Input: part model. Units: mm. Frame: model coordinates. Face numbers are marked on the shaded views. Coordinates: 2 decimals unless noted, no trailing zeros. Order: outer loops, then holes, each group sorted by start corner. A loop starts at its lowest first (then second) coordinate and runs counter-clockwise, first axis right, second up. Notation, with made-up numbers: (33.5, 37.5) -> (87.5, 37.5) arc R28 cw to (87.5, 60.5) -> close; hole circle Ø3 at (26.5, 54.25). An arc over 180 degrees is marked (long way). Write each question's results on one line, items separated by ' | '.
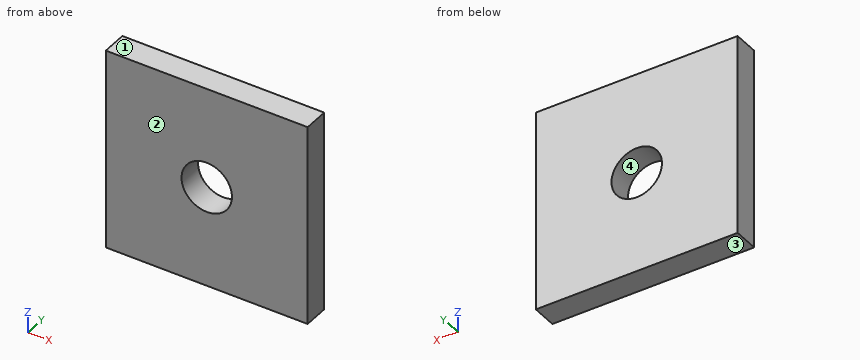
```python
from build123d import *

# Parameters (mm, degrees)
SKETCH1_W           = 76.2
SKETCH1_H           = 76.2
SKETCH1_R           = 9.525
BOSS_EXTRUDE1_DEPTH = 9.525


with BuildPart() as part:
    # Sketch1 → Boss-Extrude1 (new body)
    with BuildSketch(Plane(origin=(0, 0, 0), x_dir=(1, 0, 0), z_dir=(0, 1, 0))):
        with Locations((38.1, 38.1)):
            Rectangle(SKETCH1_W, SKETCH1_H)
        with Locations((38.1, 38.1)):
            Circle(SKETCH1_R, mode=Mode.SUBTRACT)
    extrude(amount=BOSS_EXTRUDE1_DEPTH)


solid = part.part
```
(1) Cut plane C-C, the plane y = 2. Return loops of the section in (x, z) (3 decimals), plus the area to 3 significant figures.
Return value:
outline: (0, -76.2) -> (76.2, -76.2) -> (76.2, 0) -> (0, 0) -> close; hole circle Ø19.05 at (38.1, -38.1) | area: 5,520 mm2
(2) Pin query (flat end, axial travel): P1, Ø8, axis at x = 38.5, z = -43, coming from the +Y side. Return the tip coordinate at first contact, or that it passes through.
Return value:
P1: through
(3) Line query: line 1 along X through (y, z) = (4, -38.1) (3 decimals); line 2 along Z through (x, y) = (38.1, 4.25) (3 decimals); line 3 along X through (y, z) = (6.5, -45). Output: solid intervals per line, ascending. Write a range as from..to.
Return value:
line 1: 0..28.575, 47.625..76.2 | line 2: -76.2..-47.625, -28.575..0 | line 3: 0..31.53, 44.67..76.2
(4) Cut plane B-B, the plane x = 38.1. Return loops of the section in (y, z) (3 decimals).
Return value:
outline: (0, -76.2) -> (9.525, -76.2) -> (9.525, -47.625) -> (0, -47.625) -> close; (0, -28.575) -> (9.525, -28.575) -> (9.525, 0) -> (0, 0) -> close
(5) Cut plane A-A, the plane z = -38.1. Return loops of the section in (x, y) (3 decimals), plus the area to 3 significant figures.
Return value:
outline: (0, 0) -> (28.575, 0) -> (28.575, 9.525) -> (0, 9.525) -> close; (47.625, 0) -> (76.2, 0) -> (76.2, 9.525) -> (47.625, 9.525) -> close | area: 544 mm2
(6) Mould query, pull axis Z, two halves, no side actions, for the marked faces 1, 2, 3 and 4. Classes: +Z half, -Z half, draft (parallel to the pull), parting line (faces both ways), or undercut.
Return value:
face 1: +Z half | face 2: draft | face 3: -Z half | face 4: undercut
